Geometry check sheet. Reference: drawing and pictorial views, mm from the part's lowest x, y, z. A direction names the side the tool comes from. Round coordinates to 2 decimals unless told otherwise and drop trailing zeros. Write each loop counter-clockwise with the first axis right and the second up, starting at its lowest first coordinate (ties: lowest second). Pieces come first, ordered by that corner, then holes. Notation, with made-up numbers: (73.25, 14) -> (88.25, 14) arc R21 ccw to (88.25, 23) -> close; hole circle Ø1 at (50, 10.5). An arc over 180 degrees is marked (long way). Answer as a JSON object with one key per item and string values. Group by question number.
(1) Sectioned sample at A-A on y = 31. Record the cut outline in (x, z), and give its area (3 significant figures).
(2) Sectioned sample at D-D on z = 23. Record the cut outline in (x, y), and give its area (3 significant figures).
(3) Set-up check for the marked faces 1, 2, 3 and 4: record each of +Z, -Z, +X, -X, +Y, -Y from which the full face is reachable in a straight line by a thin tool's end or side.
(4) Scan lines: L1, parallel to X at y = 5.5, z = 12 (1 decimal); L2, parallel to X at y = 24.5, z = 33; L3, parallel to Y at x = 14, z = 16. Record each from-to range of solid material in increasing order. Write a range as from..to.
(5) Gauge pin test, flat ends, axial feed: pin 1 Ø1.5 at (x, z) = (48.5, 25.5) entering from -Y; pin 2 Ø6 at (y, z) = (7.5, 25) entering from -X; pin 3 Ø5 at (x, z) = (27.5, 34.5) entering from -Y (1 decimal); pin 4 Ø8.5 at (x, z) = (69, 15) entering from +Y. Record the tip position at first contact, or that the pin passes through.
(6) Draft check along Z on the marked faces 5, 6, 7 and 8. Enter one of: released by +Z, released by -Z, zero draft, split by the parting line, or undercut.
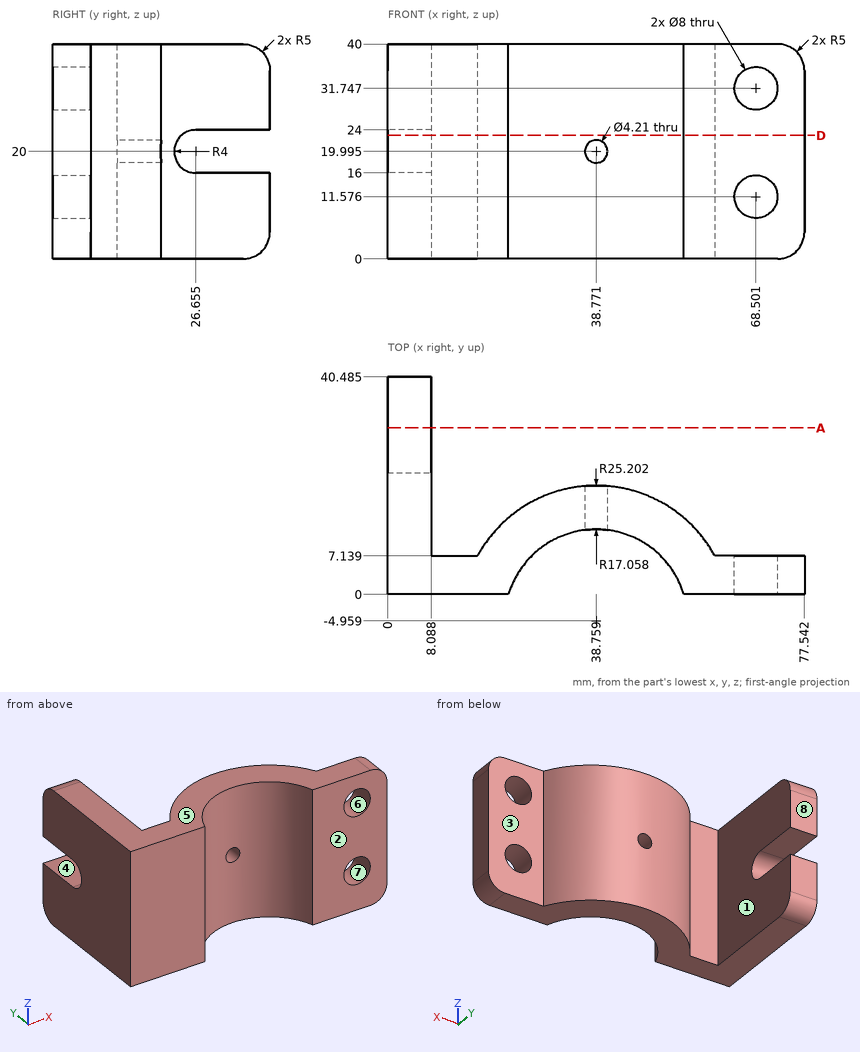
Computed values:
{
 "1": {"outline": "(0, 0) -> (8.09, 0) -> (8.09, 16) -> (0, 16) -> close; (0, 24) -> (8.09, 24) -> (8.09, 40) -> (0, 40) -> close", "area": "259 mm2"},
 "2": {"outline": "(0, 0) -> (22.44, 0) arc R17.06 cw to (55.08, 0) -> (77.54, 0) -> (77.54, 7.14) -> (60.87, 7.14) arc R25.2 ccw to (16.65, 7.14) -> (8.09, 7.14) -> (8.09, 24.01) -> (0, 24.01) -> close", "area": "812 mm2"},
 "3": {"face 1": "+Z, -Z, +Y", "face 2": "+Z, -Z, +X, -X, -Y", "face 3": "+Z, -Z, +X, +Y", "face 4": "+X, -X, +Y"},
 "4": {"L1": "0..25.3, 52.2..64.5, 72.5..77.5", "L2": "0..8.09", "L3": "0..7.14"},
 "5": {"pin 1": "y = 8.49", "pin 2": "x = 0", "pin 3": "y = 5.1", "pin 4": "y = 7.14"},
 "6": {"face 5": "released by +Z", "face 6": "undercut", "face 7": "undercut", "face 8": "zero draft"}
}
